```python
from build123d import *

# Parameters (mm, degrees)
SKETCH_1_R          = 13.9
SKETCH_1_R_2        = 2.1
SKETCH_1_W          = 50
SKETCH_1_H          = 10
SKETCH_1_R_3        = 1.6
EXTRUDE_1_DEPTH     = 10
FILLET_1_R          = 3
CUT_EXTRUDE_1_DEPTH = 10


with BuildPart() as part:
    # ｽｹｯﾁ1 → ﾎﾞｽ - 押し出し1 (new body)
    # profile 1 of 3: a face of its own
    with BuildSketch(Plane.XY):
        with Locations((0, -20)):
            Circle(SKETCH_1_R)
        with Locations((-10, -20)):
            Circle(SKETCH_1_R_2, mode=Mode.SUBTRACT)
        with Locations((10, -20)):
            Circle(SKETCH_1_R_2, mode=Mode.SUBTRACT)
    # profile 2 of 3: a face of its own
    with BuildSketch(Plane.XY):
        with BuildLine():
            Line((25, -5), (-25, -5))
            Line((-25, -5), (-11.969023725, -27.067706209))
            ThreePointArc((-11.969023725, -27.067706209), (-3.66337073, -6.591431288), (13.9, -20))
            ThreePointArc((13.9, -20), (13.408568712, -23.66337073), (11.969023725, -27.067706209))
            Line((11.969023725, -27.067706209), (25, -5))
        make_face()
    # profile 3 of 3: a face of its own
    with BuildSketch(Plane.XY):
        Rectangle(SKETCH_1_W, SKETCH_1_H)
        Circle(SKETCH_1_R_3, mode=Mode.SUBTRACT)
        with Locations((-20, 0)):
            Circle(SKETCH_1_R_3, mode=Mode.SUBTRACT)
        with Locations((20, 0)):
            Circle(SKETCH_1_R_3, mode=Mode.SUBTRACT)
    extrude(amount=EXTRUDE_1_DEPTH)

    # ﾌｨﾚｯﾄ1
    fillet_1_edges = [part.edges().sort_by_distance(p)[0] for p in [
        (-25, -5, 5),
        (-25, 5, 5),
        (25, 5, 5),
        (25, -5, 5),
    ]]
    fillet(fillet_1_edges, radius=FILLET_1_R)

    # ｽｹｯﾁ2 → ｶｯﾄ - 押し出し1 (cut)
    with BuildSketch(Plane.XY.offset(10)):
        with BuildLine():
            ThreePointArc((5.25, -20), (0, -14.75), (-5.25, -20))
            Line((-5.25, -20), (5.25, -20))
        make_face()
        with BuildLine():
            Line((5.25, -20), (-5.25, -20))
            ThreePointArc((-5.25, -20), (0, -25.25), (5.25, -20))
        make_face()
    extrude(amount=-CUT_EXTRUDE_1_DEPTH, mode=Mode.SUBTRACT)


solid = part.part
```
The model under review builds one solid part; all positions refer to its coordinate system, in mm. Give positions to 0.01 mm unless a question says otherwise; leave off trailing zeros. Order: outer loops, then holes, each group sorted by start corner. A loop starts at its lowest first (then second) coordinate and runs counter-clockwise, first axis right, second up. Notation, with made-up numbers: (52.25, 63.5) - (98.25, 63.5) arc R30 ccw to (98.25, 94.5) - close; hole circle Ø8 at (-27.5, 77). An arc over 180 degrees is marked (long way). Use CSV: the item, a comma, the result in double quotes. Start each with the question number.
Q1. To check wall thickness, follow line 1 along Y through (x, z) = (0, 5.75); line 2 along Y through (x, z) = (20, 4.75); line 3 along Y through (x, z) = (-19, 5.75). State the ranges of each line that lie inside material, in increasing order. Write a range as [from, to].
Q2. We need section D-D, the plane y = -20. Write out the cut boundary in (x, z), and give its area (3 significant figures).
Q3. We need section C-C, the plane x = 10. Write out the cut boundary in (y, z).
Q4. Clearance check with flat-ended pins moving along their axes: pin 1 Ø4 at (y, z) = (-22.5, 5) entering from -X; pin 2 Ø4 at (y, z) = (-18, 7.5) entering from +X. State where each tip first meets the part, or that it passes through.
Q5. We need section A-A, the plane z = 2.75. Write out the cut boundary in (x, y).
Q6. We need section B-B, the plane y = 0. Write out the cut boundary in (x, z), and give its area (3 significant figures).
Q7. The part is to be moulded in two halves that separate along X. For faces 1 (the cylindrical face through (-24.14, 4.1, 5.07)), 2 (the cylindrical face through (-1.27, -0.97, 4.93)), 3 (the cylindrical face through (24.1, 4.14, 5.07)), 4 (the cylindrical face through (-11.548, -18.581, 4.93)), say which applies: +X half, -X half, draft (parallel to the pull), parting line (faces both ways), or undercut.
Outcome:
1,line 1,"y = [-33.9, -25.25], [-14.75, -1.6], [1.6, 5]"
1,line 2,"y = [-13.47, -1.6], [1.6, 5]"
1,line 3,"y = [-15.16, -1.25], [1.25, 5]"
2,outline,"(-16.14, 0) - (-12.1, 0) - (-12.1, 10) - (-16.14, 10) - close; (-7.9, 0) - (-5.25, 0) - (-5.25, 10) - (-7.9, 10) - close; (5.25, 0) - (7.9, 0) - (7.9, 10) - (5.25, 10) - close; (12.1, 0) - (16.14, 0) - (16.14, 10) - (12.1, 10) - close"
2,area,"134 mm^2"
3,outline,"(-29.65, 0) - (-22.1, 0) - (-22.1, 10) - (-29.65, 10) - close; (-17.9, 0) - (5, 0) - (5, 10) - (-17.9, 10) - close"
4,pin 1,"stops at x = -15.85"
4,pin 2,"stops at x = 18.5"
5,outline,"(-25, -4.18) arc R3 ccw to (-24.58, -5.71) - (-11.97, -27.07) arc R13.9 ccw to (11.97, -27.07) - (24.58, -5.71) arc R3 ccw to (25, -4.18) - (25, 2) arc R3 ccw to (22, 5) - (-22, 5) arc R3 ccw to (-25, 2) - close; hole circle Ø3.2 at (-20, 0); hole circle Ø4.2 at (-10, -20); hole circle Ø10.5 at (0, -20); hole circle Ø3.2 at (0, 0); hole circle Ø4.2 at (10, -20); hole circle Ø3.2 at (20, 0)"
6,outline,"(-25, 0) - (-21.6, 0) - (-21.6, 10) - (-25, 10) - close; (-18.4, 0) - (-1.6, 0) - (-1.6, 10) - (-18.4, 10) - close; (1.6, 0) - (18.4, 0) - (18.4, 10) - (1.6, 10) - close; (21.6, 0) - (25, 0) - (25, 10) - (21.6, 10) - close"
6,area,"404 mm^2"
7,face 1,"-X half"
7,face 2,"undercut"
7,face 3,"+X half"
7,face 4,"undercut"
